The listing builds one solid part. Answer for the finished solid, in the listing's coordinates (mm). Face numbers are marked on the shaded views. A direction names the side the tool comes from. Coordinates: 2 decimals unless noted, no trailing zeros. Write each loop counter-clockwise with the first axis right and the second up, starting at its lowest first coordinate (ties: lowest second). Pieces come first, ordered by that corner, then holes. Notation, with made-up numbers: M 5,62.25 L 23,62.25 A17 ccw 23,88.25 Z; hole C 34.25,54 d5. An arc over 180 degrees is marked long. Answer as CSV lines item,"result".
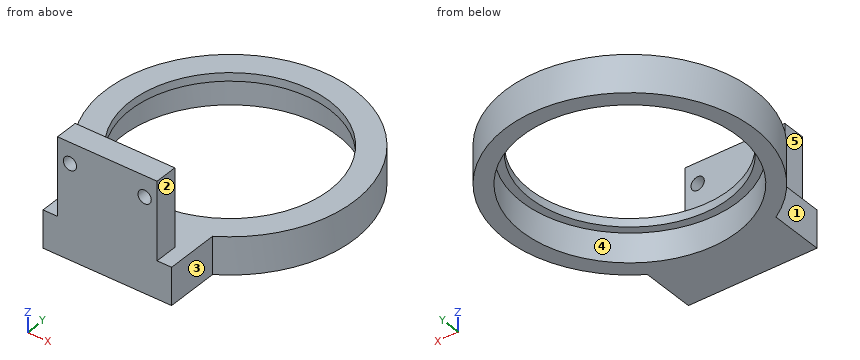
```python
from build123d import *

# Parameters (mm, degrees)
SKETCH_1_R          = 26
EXTRUDE_1_DEPTH     = 7
SKETCH_4_R          = 30
SKETCH_4_R_2        = 24
EXTRUDE_4_DEPTH     = 2
SKETCH_5_W          = 24
SKETCH_5_H          = 5
EXTRUDE_5_DEPTH     = 20.7
EXTRUDE_8_DEPTH     = 2
SKETCH_9_R          = 1.6
CUT_EXTRUDE_1_DEPTH = 6
EXTRUDE_9_DEPTH     = 0.56
SKETCH_11_R         = 1.6
CUT_EXTRUDE_2_DEPTH = 25


with BuildPart() as part:
    # 草图1 → 凸台-拉伸1 (new body)
    with BuildSketch(Plane.XY):
        with BuildLine():
            Line((-15.5, -38), (15.5, -38))
            Line((15.5, -38), (15.5, -25.685599078))
            ThreePointArc((15.5, -25.685599078), (0, 30), (-15.5, -25.685599078))
            Line((-15.5, -25.685599078), (-15.5, -38))
        make_face()
        Circle(SKETCH_1_R, mode=Mode.SUBTRACT)
    extrude(amount=EXTRUDE_1_DEPTH)

    # 草图4 → 凸台-拉伸4 (add)
    with BuildSketch(Plane.XY.offset(7)):
        Circle(SKETCH_4_R)
        Circle(SKETCH_4_R_2, mode=Mode.SUBTRACT)
    extrude(amount=EXTRUDE_4_DEPTH)

    # 草图5 → 凸台-拉伸5 (add)
    with BuildSketch(Plane.XY.offset(7)):
        with Locations((0, -35.5)):
            Rectangle(SKETCH_5_W, SKETCH_5_H)
    extrude(amount=EXTRUDE_5_DEPTH)

    # 草图6 → 凸台-拉伸8 (add)
    with BuildSketch(Plane.XY.offset(7)):
        with BuildLine():
            Line((15.5, -38), (15.5, -25.685599078))
            ThreePointArc((15.5, -25.685599078), (0, -30), (-15.5, -25.685599078))
            Line((-15.5, -25.685599078), (-15.5, -38))
            Line((-15.5, -38), (-12, -38))
            Line((-12, -38), (-12, -33))
            Line((-12, -33), (12, -33))
            Line((12, -33), (12, -38))
            Line((12, -38), (15.5, -38))
        make_face()
    extrude(amount=EXTRUDE_8_DEPTH)

    # 草图9 → 切除-拉伸1 (cut, through all)
    with BuildSketch(Plane(origin=(0, -33, 0), x_dir=(1, 0, 0), z_dir=(0, 1, 0))):
        with Locations((-9, -22.7)):
            Circle(SKETCH_9_R)
        with Locations((9, -22.7)):
            Circle(SKETCH_9_R)
    extrude(amount=-CUT_EXTRUDE_1_DEPTH, mode=Mode.SUBTRACT)

    # 草图10 → 凸台-拉伸9 (add)
    with BuildSketch(Plane.XZ.offset(38)):
        Polygon((15.5, 0), (15.5, 9), (12, 9), (12, 27.7), (-12, 27.7), (-12, 9), (-15.5, 9), (-15.5, 0), align=None)
    extrude(amount=EXTRUDE_9_DEPTH)

    # 草图11 → 切除-拉伸2 (cut)
    with BuildSketch(Plane(origin=(0, -33, 0), x_dir=(1, 0, 0), z_dir=(0, 1, 0))):
        with Locations((9, -22.7)):
            Circle(SKETCH_11_R)
        with Locations((-9, -22.7)):
            Circle(SKETCH_11_R)
    extrude(amount=-CUT_EXTRUDE_2_DEPTH, mode=Mode.SUBTRACT)


solid = part.part
```
Q1. Straight lines are drawn through the part: line 1 (X direction, y = -35.2, z = 22.7); line 2 (Z direction, x = 9, y = -34.85); line 3 (Y direction, x = 0, z = 1.5). For each, find the intervals that lie inside material, in ascending order.
Output:
line 1,"-12 to -10.6, -7.4 to 7.4, 10.6 to 12"
line 2,"0 to 21.1, 24.3 to 27.7"
line 3,"-38.56 to -26, 26 to 30"
Q2. For the marked faces 1, 2, 3, 4 and 5, determine the directions among +Z, -Z, +X, -X, +Y, -Y from which every point of the face is accessible in a straight line to the end or side of a thin tool.
Output:
face 1,"+Z, -Z, -X, -Y"
face 2,"+Z, +X, +Y, -Y"
face 3,"+Z, -Z, +X, -Y"
face 4,"-Z"
face 5,"+Z, -X, +Y, -Y"
Q3. Find section D-D (z = 2.75). Give the vertices of the cut face in (x, y), and give its area (3 significant figures).
Output:
outline,"M -15.5,-38.56 L 15.5,-38.56 L 15.5,-25.69 A30 ccw long -15.5,-25.69 Z; hole C 0,0 d52"
area,"1,010 mm2"
Q4. Find section C-C (x = 0). Give the vertices of the cut face in (y, z).
Output:
outline,"M -38.56,0 L -26,0 L -26,7 L -24,7 L -24,9 L -33,9 L -33,27.7 L -38.56,27.7 Z; M 24,7 L 26,7 L 26,0 L 30,0 L 30,9 L 24,9 Z"
Q5. Find section B-B (z = 22.7). Give the vertices of the cut face in (x, y), and give its area (3 significant figures).
Output:
outline,"M -12,-38.56 L -10.6,-38.56 L -10.6,-33 L -12,-33 Z; M -7.4,-38.56 L 7.4,-38.56 L 7.4,-33 L -7.4,-33 Z; M 10.6,-38.56 L 12,-38.56 L 12,-33 L 10.6,-33 Z"
area,"97.9 mm2"
Q6. Find section A-A (y = 0). Give the vertices of the cut face in (x, z), and give its area (3 significant figures).
Output:
outline,"M -30,0 L -26,0 L -26,7 L -24,7 L -24,9 L -30,9 Z; M 24,7 L 26,7 L 26,0 L 30,0 L 30,9 L 24,9 Z"
area,"80.0 mm2"
Q7. Flat-ended cylindrical pins translate along their axes: pin 1 Ø3.5 at (x, z) = (9, 22.7) entering from +Y; pin 2 Ø6 at (x, z) = (13.5, 11) entering from +Y; pin 3 Ø7 at (y, z) = (-33, 5.5) entering from +X; pin 4 Ø3.5 at (x, z) = (-9, 22.7) entering from -Y. Find the tip coordinate at first contact, or state that the pin passes through.
Output:
pin 1,"y = -33"
pin 2,"y = 27.81"
pin 3,"x = 15.5"
pin 4,"y = -38.56"
